For this review, use the dimensioned drawing (mm, ordinates from the lowest corner) and the shaded views. Coordinates: 2 decimals unless noted, no trailing zeros. Order: outer loops, then holes, each group sorted by start corner. A loop starts at its lowest first (then second) coordinate and runs counter-clockwise, first axis right, second up. Notation, with made-up numbers: M 84.25,-12.75 L 135.25,-12.75 A12 cw 135.25,3.25 Z; hole C -38.75,-32.75 d9. An arc over 180 degrees is marked long. Use CSV: the item, a comma, the result in double quotes.
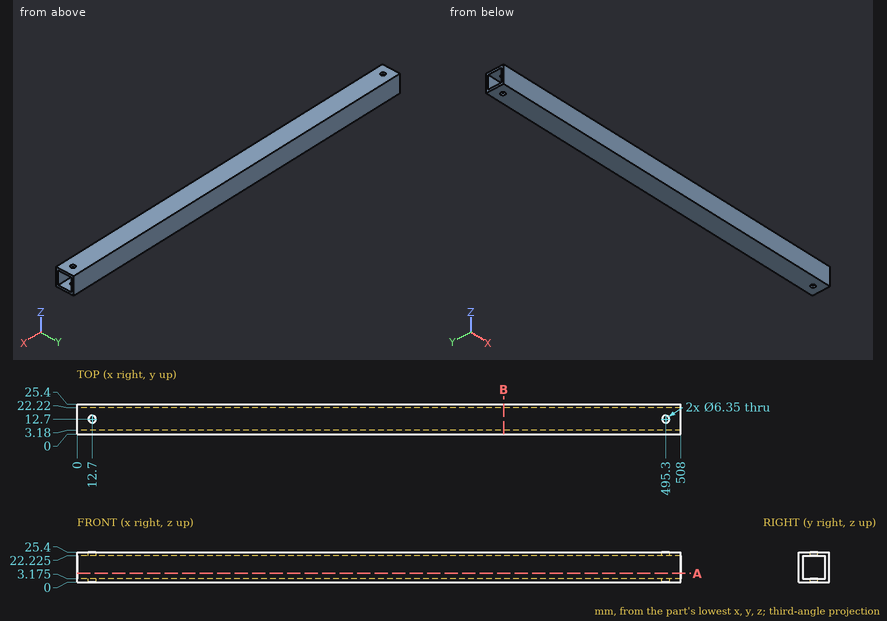
Item 1: To check wall thickness, follow line 1 along Z through (x, y) = (318, 6) (1 decimal); line 2 along Y through (x, z) = (12.7, 24.1) (1 decimal); line 3 along Y through (x, z) = (404, 8). State the ranges of each line that lie inside material, in increasing order. Write a range as [from, to].
Solutions:
line 1,"[0, 3.2], [22.2, 25.4]"
line 2,"[0, 9.5], [15.9, 25.4]"
line 3,"[0, 3.18], [22.22, 25.4]"
Item 2: Add section A-A on z = 7.5. State the section outline as (x, y) points, and give its area (3 significant figures).
Solutions:
outline,"M 0,0 L 508,0 L 508,3.18 L 0,3.18 Z; M 0,22.22 L 508,22.22 L 508,25.4 L 0,25.4 Z"
area,"3,230 mm^2"
Item 3: Add section B-B on x = 359. State the section outline as (y, z) points (1 decimal).
Solutions:
outline,"M 0,0 L 25.4,0 L 25.4,25.4 L 0,25.4 Z; hole M 3.2,3.2 L 22.2,3.2 L 22.2,22.2 L 3.2,22.2 Z"
Item 4: Clearance check with a flat-ended pin moving along its axis: pin 1 Ø4 at (x, y) = (495.3, 12.7) entering from +Z. State where the tip first meets the part, or that it passes through.
Solutions:
pin 1,"through"
